from build123d import *

# Parameters (mm, degrees)
SKETCH_W          = 72
SKETCH_H          = 41
PAD_DEPTH         = 2
SKETCH001_W       = 40.3
SKETCH001_H       = 21
PAD001_DEPTH      = 2
SKETCH002_W       = 7.5
SKETCH002_H       = 19.5
SKETCH002_R       = 2.15
PAD002_DEPTH      = 2.5
PAD002_DEPTH_BACK = -2
POCKET_DEPTH      = 173.977743
FILLET_R          = 1


with BuildPart() as part:
    # Sketch → Pad (new body)
    with BuildSketch(Plane.XY):
        Rectangle(SKETCH_W, SKETCH_H)
    extrude(amount=PAD_DEPTH)

    # Sketch001 (on Face2 of Pad) → Pad001 (join)
    with BuildSketch(Plane.XZ.offset(20.5)):
        with Locations((0, 12.5)):
            Rectangle(SKETCH001_W, SKETCH001_H)
    extrude(amount=-PAD001_DEPTH)

    # Sketch002 (on DatumPlane) → Pad002 (join, two sides)
    with BuildSketch(Plane(origin=(0, 8.1, 0), x_dir=(-1, 0, 0), z_dir=(0, 1, 0))) as pad002_sk:
        with Locations((23.9, 11.75)):
            Rectangle(SKETCH002_W, SKETCH002_H)
        with Locations((24.3, 17.5)):
            Circle(SKETCH002_R, mode=Mode.SUBTRACT)
        with Locations((24.3, 8)):
            Circle(SKETCH002_R, mode=Mode.SUBTRACT)
        with Locations((-23.9, 11.75)):
            Rectangle(SKETCH002_W, SKETCH002_H)
        with Locations((-24.3, 17.5)):
            Circle(SKETCH002_R, mode=Mode.SUBTRACT)
        with Locations((-24.3, 8)):
            Circle(SKETCH002_R, mode=Mode.SUBTRACT)
    extrude(amount=-PAD002_DEPTH)
    extrude(pad002_sk.sketch, amount=-PAD002_DEPTH_BACK)

    # Sketch003 (on Face5 of Pad002) → Pocket (cut, through all)
    with BuildSketch(Plane.XY.offset(2)):
        with BuildLine():
            ThreePointArc((33.475, 16.5), (31.825, 18.15), (30.175, 16.5))
            Line((30.175, 16.5), (30.175, -16.5))
            ThreePointArc((30.175, -16.5), (31.825, -18.15), (33.475, -16.5))
            Line((33.475, 16.5), (33.475, -16.5))
        make_face()
    pocket = extrude(amount=-POCKET_DEPTH, mode=Mode.SUBTRACT)

    # Mirrored: Pocket across YZ
    add(pocket.mirror(Plane.YZ), mode=Mode.SUBTRACT)

    # Fillet
    fillet_edges = [part.edges().sort_by_distance(p)[0] for p in [
        (-20.15, 7.85, 2),
        (-23.9, 5.6, 2),
        (-27.65, 7.85, 2),
        (-23.9, 10.1, 2),
        (-20.15, 7.85, 21.5),
        (-27.65, 7.85, 21.5),
        (20.15, 7.85, 21.5),
        (27.65, 7.85, 21.5),
        (27.65, 7.85, 2),
        (23.9, 5.6, 2),
        (23.9, 10.1, 2),
        (20.15, 7.85, 2),
        (20.15, -19.5, 2),
        (0, -18.5, 2),
        (-20.15, -19.5, 2),
    ]]
    fillet(fillet_edges, radius=FILLET_R)


solid = part.part
Design review of the part built by this model. Coordinates are the model's own, in mm. A direction names the side the tool comes from. Coordinates: 2 decimals unless noted, no trailing zeros. Order: outer loops, then holes, each group sorted by start corner. A loop starts at its lowest first (then second) coordinate and runs counter-clockwise, first axis right, second up. Notation, with made-up numbers: M 87.25,-2 L 103.25,-2 A16 ccw 103.25,4 Z; hole C 30.25,-10 d11. An arc over 180 degrees is marked long. Use a Markdown table: item, result.
(1) For faces 4 (the cylindrical face through (31.86, 18.15, 1.01)), 5 (the flat face through (27.65, 8, 12)), 6 (the flat face through (24, 10.1, 12)), 7 (the flat face through (-20.15, 8, 12)), list the 3-axis set-ups (+Z, -Z, +X, -X, +Y, -Y) from which the entire face can be reached by the end or side of a thin tool; tool diameter is ignored.
Worked answers:
| item | result |
|---|---|
| face 4 | +Z, -Z |
| face 5 | +Z, +X, +Y, -Y |
| face 6 | +Z, +X, -X, +Y |
| face 7 | +Z, +Y |
(2) Add section C-C (z = 4). Give the boundary of the cut face in (x, y).
Worked answers:
| item | result |
|---|---|
| outline | M -27.65,5.6 L -20.15,5.6 L -20.15,10.1 L -27.65,10.1 Z; M -20.15,-20.5 L 20.15,-20.5 L 20.15,-18.5 L -20.15,-18.5 Z; M 20.15,5.6 L 27.65,5.6 L 27.65,10.1 L 20.15,10.1 Z |
(3) Wall thickness on probe 1 along Z at (x, y) = (-24, 7); probe 2 along Z at (x, y) = (-5, 2.5); probe 3 along Y at (x, z) = (14, 5): over which ranges is each line inside the solid? List them lowest first.
Worked answers:
| item | result |
|---|---|
| probe 1 | z = 0 to 5.87, 10.13 to 15.37, 19.63 to 21.5 |
| probe 2 | z = 0 to 2 |
| probe 3 | y = -20.5 to -18.5 |
(4) Add section D-D (x = -24.3). Give the boundary of the cut face in (y, z).
Worked answers:
| item | result |
|---|---|
| outline | M -20.5,0 L 20.5,0 L 20.5,2 L 11.1,2 A1 cw 10.1,3 L 10.1,5.85 L 5.6,5.85 L 5.6,3 A1 cw 4.6,2 L -20.5,2 Z; M 5.6,10.15 L 10.1,10.15 L 10.1,15.35 L 5.6,15.35 Z; M 5.6,19.65 L 10.1,19.65 L 10.1,21.5 L 5.6,21.5 Z |
(5) Draft analysis for pull direction Y (two halves, no side actions). For faces 1 (the flat face through (33.475, 0, 1)), 2 (the flat face through (24, 8, 21.5)), 3 (the flat face through (-1, 20.5, 1)), state which applies: released by +Y, released by -Y, zero draft, split by the parting line, or undercut.
Worked answers:
| item | result |
|---|---|
| face 1 | undercut |
| face 2 | zero draft |
| face 3 | released by +Y |
(6) Add section A-A (y = 7). Count the separate pieces of the cut face and the enclosed holes in it, then the cut area to 3 significant figures.
Worked answers:
| item | result |
|---|---|
| separate pieces | 3 |
| enclosed holes | 4 |
| area | 365 mm2 |
(7) For P1, Ø4, axis at x = -9, y = 7, coming from the +Z side; P2, Ø2, axis at y = -20, z = 13.5, coming from the -X side; P3, Ø5, axis at x = -24.3, z = 8, coming from the -Y side; P4, Ø5, axis at y = 3, z = 11.5, coming from the +X side, all flat-tipped, find the tip position at first contact; note any pin that passes through.
Worked answers:
| item | result |
|---|---|
| P1 | stops at z = 2 |
| P2 | stops at x = -20.15 |
| P3 | stops at y = 5.6 |
| P4 | passes through |
(8) Add section B-B (z = 17.5). Give the boundary of the cut face in (x, y).
Worked answers:
| item | result |
|---|---|
| outline | M -27.65,5.6 L -26.45,5.6 L -26.45,10.1 L -27.65,10.1 Z; M -22.15,5.6 L -20.15,5.6 L -20.15,10.1 L -22.15,10.1 Z; M -20.15,-20.5 L 20.15,-20.5 L 20.15,-18.5 L -20.15,-18.5 Z; M 20.15,5.6 L 22.15,5.6 L 22.15,10.1 L 20.15,10.1 Z; M 26.45,5.6 L 27.65,5.6 L 27.65,10.1 L 26.45,10.1 Z |
